```python
from build123d import *

# Parameters (mm, degrees)
F1_DEPTH = 10
F2_DEPTH = 3
F3_R     = 8
F4_D     = 14
F6_D     = 2.5


# Not quite as in the source:
# - a fillet or chamfer that OpenCascade refuses, or shapes differently, is made with other operations: its cross-section is extruded or revolved along the edge and cut away or added


with BuildPart() as f1:
    # F0 (on Top) → F1 (new body)
    with BuildSketch(Plane.XY):
        with BuildLine():
            ThreePointArc((8.4283100441, 1.101630519), (-0.5519803552, 8.482058576), (-8.5, 0))
            Line((-8.5, 0), (8.4283100441, 0))
            Line((8.4283100441, 0), (8.4283100441, 1.101630519))
        make_face()
        with BuildLine():
            Line((8.4283100441, 0), (-8.5, 0))
            ThreePointArc((-8.5, 0), (0, -8.5), (8.5, 0))
            ThreePointArc((8.5, 0), (8.482058576, 0.5519803552), (8.4283100441, 1.101630519))
            Line((8.4283100441, 1.101630519), (8.4283100441, 0))
        make_face()
    extrude(amount=F1_DEPTH)

    # F0 (on Top) → F2 (join)
    with BuildSketch(Plane.XY):
        with BuildLine():
            Line((-8.5, 26.0569844395), (-8.5, 0))
            ThreePointArc((-8.5, 0), (-0.5519803552, 8.482058576), (8.4283100441, 1.101630519))
            Line((8.4283100441, 1.101630519), (8.4283100441, 26.0569844395))
            Line((8.4283100441, 26.0569844395), (-8.5, 26.0569844395))
        make_face()
    extrude(amount=F2_DEPTH)

    # F3
    f3_edges = [f1.edges().sort_by_distance(p)[0] for p in [
        (-8.5, 26.056984, 1.5),
        (8.42831, 26.056984, 1.5),
    ]]
    fillet(f3_edges, radius=F3_R)

    # F4 (through all)
    with Locations(Plane(origin=(0, 0, 0), x_dir=(1, 0, 0), z_dir=(0, 0, -1))):
        with Locations((0, 0)):
            Hole(F4_D / 2)

    # F5: chamfer of 1 on 1 edges, made by hand

    # F5_s1 → F5_t2 (revolve, cut)
    with BuildSketch(Plane.XZ):
        Polygon((-8.5, 9), (-7.5, 10), (-8.5, 10), align=None)
    revolve(axis=Axis((0, 0, 10), (0, 0, 1)), mode=Mode.SUBTRACT)

    # F6 (through all)
    with Locations(Plane(origin=(0, 0, 0), x_dir=(1, 0, 0), z_dir=(0, 0, -1))):
        with Locations((0, -21), (0, -13)):
            Hole(F6_D / 2)


solid = f1.part
```
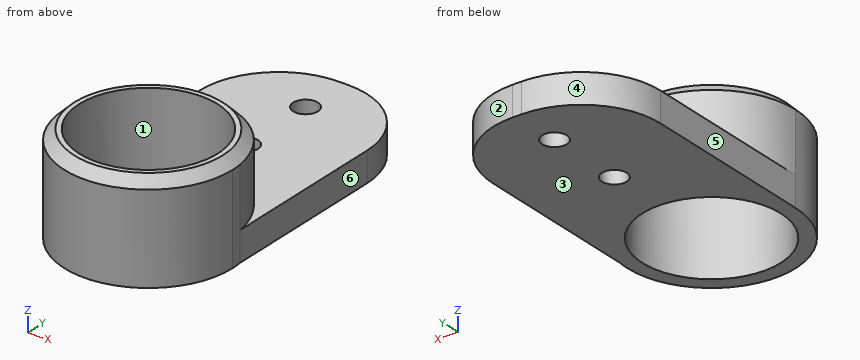
Design review of the part built by this model. Coordinates are the model's own, in mm. Face numbers are marked on the shaded views. A direction names the side the tool comes from. Round coordinates to 2 decimals unless told otherwise and drop trailing zeros. Order: outer loops, then holes, each group sorted by start corner. A loop starts at its lowest first (then second) coordinate and runs counter-clockwise, first axis right, second up. Notation, with made-up numbers: (-36, -14) - (-16, -14) arc R21 cw to (-16, 1) - close; hole circle Ø3 at (32, 88.5). An arc over 180 degrees is marked (long way). Return JSON: item names as keys, results as strings.
Q1. Consider section B-B on y = 13. Write out the cut boundary in (x, z), plus the area to 3 significant figures.
Computed values:
{"outline": "(-8.5, 0) - (-1.25, 0) - (-1.25, 3) - (-8.5, 3) - close; (1.25, 0) - (8.43, 0) - (8.43, 3) - (1.25, 3) - close", "area": "43.3 mm2"}
Q2. Consider section D-D on z = 6. Write out the cut boundary in (x, y), plus the area to 3 significant figures.
Computed values:
{"outline": "circle Ø17 at (0, 0); hole circle Ø14 at (0, 0)", "area": "73.0 mm2"}
Q3. For pin 1 Ø4 at (x, y) = (-2.5, 19.5) entering from +Z; pin 2 Ø1.5 at (y, z) = (21, 1.5) entering from +X; pin 3 Ø3 at (y, z) = (12.5, 4) entering from +X, all flat-tipped, find the tip position at first contact; note any pin that passes through.
Computed values:
{"pin 1": "stops at z = 3", "pin 2": "stops at x = 8.12", "pin 3": "stops at x = 8.43"}
Q4. Consider section A-A on x = 0. Write out the cut boundary in (y, z), plus the area to 3 significant figures.
Computed values:
{"outline": "(-8.5, 0) - (-7, 0) - (-7, 10) - (-7.5, 10) - (-8.5, 9) - close; (7, 0) - (11.75, 0) - (11.75, 3) - (8.5, 3) - (8.5, 9) - (7.5, 10) - (7, 10) - close; (14.25, 0) - (19.75, 0) - (19.75, 3) - (14.25, 3) - close; (22.25, 0) - (26.06, 0) - (26.06, 3) - (22.25, 3) - close", "area": "66.7 mm2"}
Q5. Consider section C-C on z = 2.5. Write out the cut boundary in (x, y), plus the area to 3 significant figures.
Computed values:
{"outline": "(-8.5, 0) arc R8.5 ccw (long way) to (8.43, 1.1) - (8.43, 18.06) arc R8 ccw to (0.43, 26.06) - (-0.5, 26.06) arc R8 ccw to (-8.5, 18.06) - close; hole circle Ø14 at (0, 0); hole circle Ø2.5 at (0, 13); hole circle Ø2.5 at (0, 21)", "area": "363 mm2"}
Q6. The part is to be moulded in two halves that separate along X. For the marked faces 1, 2, 3 and 4, say which applies: pulls with the +X half, pulls with the -X half, needs draft (parallel to the pull), parting line crosses it, or undercut.
Computed values:
{"face 1": "undercut", "face 2": "pulls with the +X half", "face 3": "needs draft", "face 4": "pulls with the -X half"}
Q7. Wall thickness on L1, parallel to Y at x = 0, z = 2.2; L2, parallel to Y at x = 0, z = 5.5; L3, parallel to Z at x = 2.25, y = 21: over which ranges is each line inside the solid? List them lowest first. Write a range as [from, to].
Computed values:
{"L1": "y = [-8.5, -7], [7, 11.75], [14.25, 19.75], [22.25, 26.06]", "L2": "y = [-8.5, -7], [7, 8.5]", "L3": "z = [0, 3]"}
Q8. Machinability: for the marked faces 5 and 6, which of the approach directions +Z, -Z, +X, -X, +Y, -Y give a long, thin tool a straight path to every point of the face, cutting with its end or side? Answer none if there is none.
Computed values:
{"face 5": "+Z, -Z, -X, +Y, -Y", "face 6": "+Z, -Z, +X, +Y"}
